The drawing under review shows one solid part. Ordinate dimensions are in mm from its lowest x, y, z. A direction names the side the tool comes from. Round coordinates to 2 decimals unless told otherwise and drop trailing zeros. Write each loop counter-clockwise with the first axis right and the second up, starting at its lowest first coordinate (ties: lowest second). Pieces come first, ordered by that corner, then holes. Notation, with made-up numbers: (75, 29.25) -> (119, 29.25) arc R27 cw to (119, 63.25) -> close; hole circle Ø10 at (45, 17.25). An arc over 180 degrees is marked (long way). Use CSV: the item, a comma, the result in double quotes. Start each with the question number.
1) Take a section at B-B, the plane z = 4.6. Give the boundary of the cut face in (x, y).
2) Machinability: for the marked faces 4, 5 and 6, which of the approach directions +Z, -Z, +X, -X, +Y, -Y give a long, thin tool a straight path to every point of the face, cutting with its end or side? Answer none if there is none.
3) Take a section at D-D, the plane y = 2. Give the boundary of the cut face in (x, z), then the cut area to 3 significant figures.
4) Take a section at A-A, the plane z = 1.25. Give the boundary of the cut face in (x, y), then the cut area to 3 significant figures.
5) Take a section at C-C, the plane x = 8. Give the boundary of the cut face in (y, z).
6) For pin 1 Ø0.5 at (y, z) = (5, 0.5) entering from -X, flat-tipped, find the tip position at first contact; note if it passes through.
7) Wall thickness on probe 1 along Y at (x, z) = (12.25, 1.5); probe 2 along Z at (x, y) = (8, 5.25); probe 3 along Z at (x, y) = (8, 3.5): over which ranges is each line inside the solid? List them lowest first. Write a range as [from, to].
8) Mouldability with a two-part tool opening along X and no side actions: class the marked faces 1, 2 and 3 as released by +X, released by -X, zero draft, split by the parting line, or undercut.
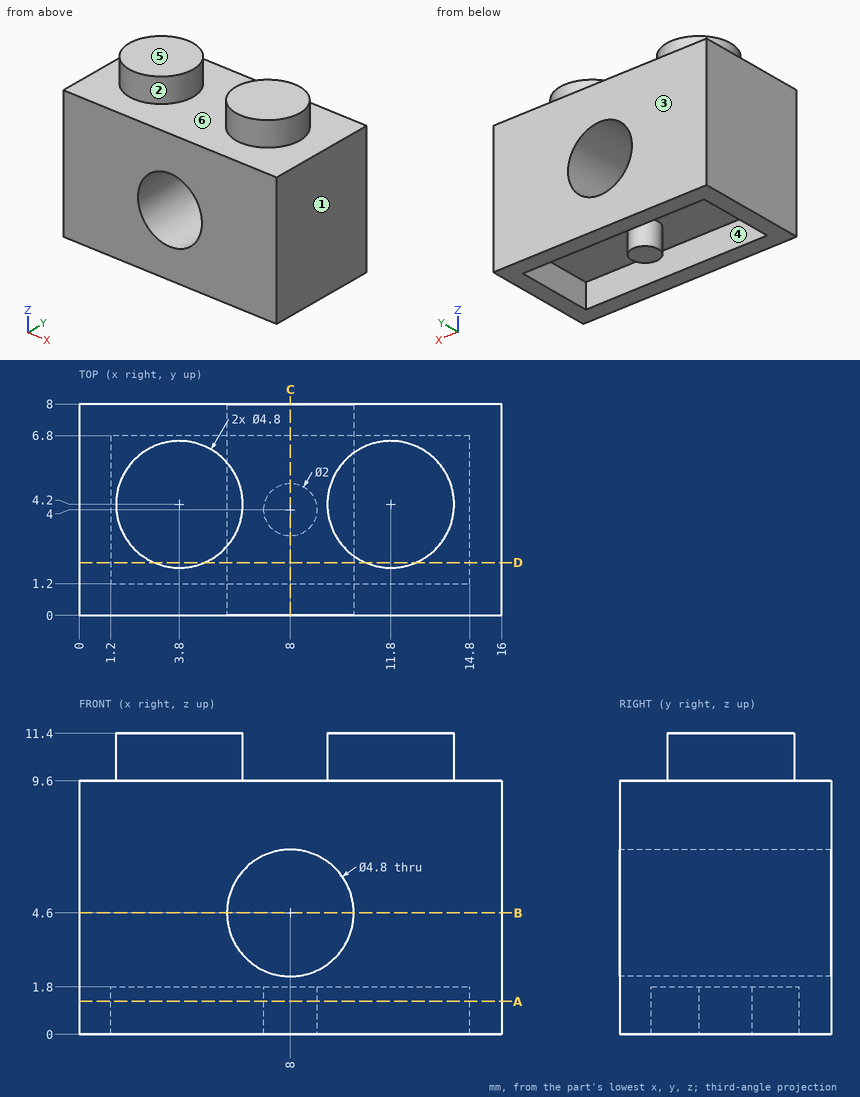
Values found:
1,outline,"(0, 0) -> (5.6, 0) -> (5.6, 8) -> (0, 8) -> close; (10.4, 0) -> (16, 0) -> (16, 8) -> (10.4, 8) -> close"
2,face 4,"-Z"
2,face 5,"+Z, +X, -X, +Y, -Y"
2,face 6,"+Z"
3,outline,"(0, 0) -> (1.2, 0) -> (1.2, 1.8) -> (14.8, 1.8) -> (14.8, 0) -> (16, 0) -> (16, 9.6) -> (12.76, 9.6) -> (12.76, 11.4) -> (10.84, 11.4) -> (10.84, 9.6) -> (4.76, 9.6) -> (4.76, 11.4) -> (2.84, 11.4) -> (2.84, 9.6) -> (0, 9.6) -> close; hole circle Ø4.8 at (8, 4.6)"
3,area,"118 mm²"
4,outline,"(0, 0) -> (16, 0) -> (16, 8) -> (0, 8) -> close; circle Ø2 at (8, 4); hole (1.2, 1.2) -> (14.8, 1.2) -> (14.8, 6.8) -> (1.2, 6.8) -> close"
4,area,"55.0 mm²"
5,outline,"(0, 0) -> (1.2, 0) -> (1.2, 1.8) -> (3, 1.8) -> (3, 0) -> (5, 0) -> (5, 1.8) -> (6.8, 1.8) -> (6.8, 0) -> (8, 0) -> (8, 2.2) -> (0, 2.2) -> close; (0, 7) -> (8, 7) -> (8, 9.6) -> (0, 9.6) -> close"
6,pin 1,"x = 0"
7,probe 1,"[0, 1.2], [6.8, 8]"
7,probe 2,"[1.8, 2.2], [7, 9.6]"
7,probe 3,"[0, 2.2], [7, 9.6]"
8,face 1,"released by +X"
8,face 2,"undercut"
8,face 3,"zero draft"
